from build123d import *

# Parameters (mm, degrees)
SKETCH_R             = 20
SKETCH_R_2           = 18.5
PAD_DEPTH            = 240
SKETCH007_R          = 1
POCKET_DEPTH         = 20.001
POCKET_DEPTH_BACK    = 20.001
SKETCH008_R          = 1
POCKET001_DEPTH      = 20.001
POCKET001_DEPTH_BACK = -20.001


with BuildPart() as part:
    # Sketch → Pad (new body)
    with BuildSketch(Plane.XY):
        Circle(SKETCH_R)
        Circle(SKETCH_R_2, mode=Mode.SUBTRACT)
    extrude(amount=PAD_DEPTH)

    # Sketch007 → Pocket (cut, two sides)
    with BuildSketch(Plane.YZ) as pocket_sk:
        with Locations((0, 96)):
            Circle(SKETCH007_R)
        with BuildLine():
            Line((1, 0), (22, 0))
            Line((22, 0), (22, 25))
            Line((22, 25), (3, 25))
            ThreePointArc((3, 25), (1.585786, 24.414214), (1, 23))
            Line((1, 23), (1, 0))
        make_face()
        with BuildLine():
            Line((1, 240), (22, 240))
            Line((22, 240), (22, 215))
            Line((22, 215), (3, 215))
            ThreePointArc((1, 217), (1.585786, 215.585786), (3, 215))
            Line((1, 217), (1, 240))
        make_face()
    extrude(amount=POCKET_DEPTH, mode=Mode.SUBTRACT)
    extrude(pocket_sk.sketch, amount=-POCKET_DEPTH_BACK, mode=Mode.SUBTRACT)

    # Sketch008 → Pocket001 (cut, two sides)
    with BuildSketch(Plane.XZ) as pocket001_sk:
        with Locations((0, 96)):
            Circle(SKETCH008_R)
    extrude(amount=-POCKET001_DEPTH, mode=Mode.SUBTRACT)
    extrude(pocket001_sk.sketch, amount=-POCKET001_DEPTH_BACK, mode=Mode.SUBTRACT)


solid = part.part
Build history of the part. All positions in model axes, mm. A direction names the side the tool comes from. Round coordinates to 2 decimals unless told otherwise and drop trailing zeros. Loops run counter-clockwise (first coordinate to the right, second up) from the corner with the lowest first, then second, coordinate; pieces in that order, holes last. Notation, with made-up numbers: (84.5, -30) -> (130.5, -30) arc R21 ccw to (130.5, -22) -> close; hole circle Ø8 at (-11.5, 70). An arc over 180 degrees is marked (long way). One line per item, written item: value. Start each with the question number.
Q1. Drop flat-ended pins along their axis: pin 1 Ø8 at (x, z) = (-5, 72.5) entering from +Y (3 decimals); pin 2 Ø2 at (y, z) = (-5, 66.5) entering from +X; pin 3 Ø0.8 at (x, z) = (19.5, 227.5) entering from +Y; pin 4 Ø2.5 at (y, z) = (0, 96) entering from +X. Give the stop position or say it passes through.
Q2. 3-axis set-ups, long thin cutter, end or side, ignore diameter. For faces 1 (the face through (0, 19, 215)), 2 (the face through (0, -19, 240)): which of +Z, -Z, +X, -X, +Y, -Y reach the whole face in a straight line?
Q3. Probe line 1 along Z through (x, y) = (18.95, 0); line 2 along Z through (x, y) = (0, 19); line 3 along X through (y, z) = (0, 94.5). List the from-to ranges inside material, lowest first.
Q4. Two-plate mould, pull along X, no slides. Class faces 3 (the face through (-4.336, -19.524, 118.32)), 4 (the face through (0, 19, 25)), 5 (the face through (-4.01, -18.06, 118.32)): released by +X, released by -X, zero draft, split by the parting line, or undercut.
Q5. Cut at A-A on x = 15. List the corners of the cut face in (y, z).
Q6. Cut at B-B on y = -8. List the corners of the cut face in (x, z), plus the area to 3 significant figures.
Q7. Cut at C-C on z = 57. List the corners of the cut face in (x, y), plus the area to 3 significant figures.
Computed:
1. pin 1: y = 19.975
1. pin 2: x = 19.6
1. pin 3: y = 1
1. pin 4: x = 20
2. face 1: +Z, +X, -X, +Y
2. face 2: +Z, +X, -X, +Y, -Y
3. line 1: 0 to 95, 97 to 240
3. line 2: 25 to 95, 97 to 215
3. line 3: -20 to -18.5, 18.5 to 20
4. face 3: split by the parting line
4. face 4: zero draft
4. face 5: undercut
5. outline: (-13.23, 0) -> (-10.83, 0) -> (-10.83, 240) -> (-13.23, 240) -> close; (10.83, 25) -> (13.23, 25) -> (13.23, 215) -> (10.83, 215) -> close
6. outline: (-18.33, 0) -> (-16.68, 0) -> (-16.68, 240) -> (-18.33, 240) -> close; (16.68, 0) -> (18.33, 0) -> (18.33, 240) -> (16.68, 240) -> close
6. area: 792 mm²
7. outline: circle Ø40 at (0, 0); hole circle Ø37 at (0, 0)
7. area: 181 mm²
